Work out the finished part from the listing and answer in its coordinate system (mm). Face numbers are marked on the shaded views. Round coordinates to 2 decimals unless told otherwise and drop trailing zeros. Order: outer loops, then holes, each group sorted by start corner. A loop starts at its lowest first (then second) coordinate and runs counter-clockwise, first axis right, second up. Notation, with made-up numbers: M 76.25,20.25 L 92.25,20.25 A23 ccw 92.25,45.25 Z; hole C 14.5,-25 d10. An arc over 180 degrees is marked long. Return JSON: item names as keys, results as strings.
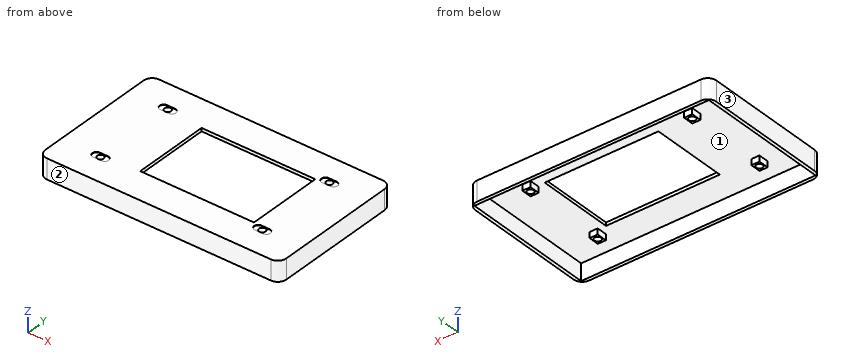
Autodesk Inventor part; units mm, degrees
ref_plane "Work Plane4" through (92.935, -15.405, 0) normal (0, 0, 1) x (1, 0, 0)
ref_plane "Work Plane5" through (-62.51, -33.015, -8.55) normal (0, 0, 1) x (1, 0, 0)
ref_plane "YZ Plane" through (0, 0, 0) normal (1, 0, 0) x (0, 1, 0)
ref_plane "Work Plane3" through (32.97, 21.365, 7.071) normal (0, 0, 1) x (1, 0, 0)
sketch "Sketch3" plane through (32.97, 21.365, 7.071) normal (0, 0, 1) x (1, 0, 0)
  line L0 (93.98, -54.61) -> (-93.98, -54.61)
  line L1 (-93.98, -54.61) -> (-93.98, 54.61)
  line L2 (-93.98, 54.61) -> (93.98, 54.61)
  line L3 (93.98, 54.61) -> (93.98, -54.61)
  line L4 (93.98, -54.61) -> (-93.98, 54.61) construction
  line L5 (-93.98, -54.61) -> (93.98, 54.61) construction
  line L6 (83.1, 48.8) -> (83.1, -50.3)
  line L7 (-81.6, 50.3) -> (81.6, 50.3)
  line L8 (-32.5, -25) -> (-32.5, 25)
  line L9 (52.4242, 25) -> (52.4242, -25)
  line L10 (49.4242, -28) -> (-29.5, -28)
  line L11 (-29.5, 28) -> (49.4242, 28)
  line L12 (-34.405, 29.905) -> (54.3292, 29.905)
  line L13 (54.3292, 29.905) -> (54.3292, -29.905)
  line L14 (54.3292, -29.905) -> (-34.405, -29.905)
  line L15 (-34.405, -29.905) -> (-34.405, 29.905)
  line L16 (49.4242, 28) -> (-29.5, 28)
  line L17 (-32.5, 25) -> (-32.5, -25)
  line L18 (49.4242, -28) -> (-29.5, -28)
  point P0 (-56.9284, 33.08)
  dimension "d6" = 187.96
  dimension "d7" = 109.22
  dimension "d8" = 4.31
  dimension "d9" = 10.88
  dimension "d55" = 1.905
  dimension "d56" = 1.905
  dimension "d57" = 1.905
  dimension "d58" = 1.905
extrude "Extrusion2" add sketch "Sketch3" against normal blind 2.54
sketch "Sketch5" plane through (32.97, 21.365, 7.071) normal (0, 0, 1) x (1, 0, 0)
  circle A0 centre (-63.1, 32.8) radius 1.5
  circle A1 centre (-63.1, -32.8) radius 1.5
  circle A2 centre (63.1, 32.8) radius 1.5
  circle A3 centre (63.1, 32.8) radius 1.5
  circle A4 centre (63.1, 32.8) radius 1.5
  circle A5 centre (63.1, 32.8) radius 1.5
  circle A6 centre (63.1, -32.8) radius 1.5
  line L0 (-59.965, 36.77) -> (-59.965, 28.83)
  line L1 (-59.965, 36.77) -> (-66.235, 36.77)
  line L2 (-66.235, 36.77) -> (-66.235, 28.83)
  line L3 (-59.965, 28.83) -> (-66.235, 28.83)
  circle A7 centre (-63.1, 32.8) radius 1.5
  line L4 (25.03, 27.635) -> (32.97, 27.635)
  line L5 (25.03, 27.635) -> (25.03, 21.365)
  line L6 (25.03, 21.365) -> (32.97, 21.365)
  line L7 (32.97, 27.635) -> (32.97, 21.365)
  circle A8 centre (29, 24.5) radius 1.25
  line L8 (-59.965, -28.83) -> (-59.965, -36.77)
  line L9 (-59.965, -28.83) -> (-66.235, -28.83)
  line L10 (-66.235, -28.83) -> (-66.235, -36.77)
  line L11 (-59.965, -36.77) -> (-66.235, -36.77)
  circle A9 centre (-63.1, -32.8) radius 1.5
  line L12 (66.235, -28.83) -> (66.235, -36.77)
  line L13 (66.235, -28.83) -> (59.965, -28.83)
  line L14 (59.965, -28.83) -> (59.965, -36.77)
  line L15 (66.235, -36.77) -> (59.965, -36.77)
  circle A10 centre (63.1, -32.8) radius 1.5
  line L16 (66.235, 36.77) -> (66.235, 28.83)
  line L17 (66.235, 36.77) -> (59.965, 36.77)
  line L18 (59.965, 36.77) -> (59.965, 28.83)
  line L19 (66.235, 28.83) -> (59.965, 28.83)
  circle A11 centre (63.1, 32.8) radius 1.5
  point P0 (-32.97, -21.365)
sketch "Sketch4" plane through (32.97, 21.365, 7.071) normal (0, 0, 1) x (1, 0, 0)
  circle A0 centre (-63.1, 32.8) radius 1.5
  circle A1 centre (-63.1, -32.8) radius 1.5
  circle A2 centre (63.1, -32.8) radius 1.5
  circle A3 centre (63.1, 32.8) radius 1.5
  circle A4 centre (-63.1, 32.8) radius 2.54
  circle A5 centre (63.1, 32.8) radius 2.54
  circle A6 centre (-63.1, -32.8) radius 2.54
  circle A7 centre (63.1, -32.8) radius 2.54
  point P0 (-32.97, -21.365)
  dimension "d12" = 5.08
ref_plane "Work Plane4" through (92.935, -15.405, 0) normal (0, 0, 1) x (1, 0, 0)
extrude "Extrusion3" add sketch "Sketch5" against normal up to surface (7.071 mm away) contours A2 | A6 | L0 L3 L2 L1 | L8 L11 L10 L9 | L12 L15 L14 L13 | L16 L19 L18 L17
extrude "Extrusion4" cut sketch "Sketch4" against normal up to surface (7.071 mm away) contours A0 | A1 | A2 | A3 | A4 | A5 | A6 | A7
ref_plane "Work Plane5" through (-62.51, -33.015, -8.55) normal (0, 0, 1) x (1, 0, 0)
sketch "Sketch7" plane through (32.97, 21.365, 4.531) normal (0, 0, -1) x (-1, 0, 0)
  line L0 (-91.44, 52.07) -> (91.44, 52.07)
  line L1 (91.44, 52.07) -> (91.44, -52.07)
  line L2 (91.44, -52.07) -> (-91.44, -52.07)
  line L3 (-91.44, -52.07) -> (-91.44, 52.07)
  line L4 (-91.44, 52.07) -> (91.44, -52.07) construction
  line L5 (91.44, 52.07) -> (-91.44, -52.07) construction
  line L6 (-93.98, -54.61) -> (93.98, -54.61)
  line L7 (93.98, -54.61) -> (93.98, 54.61)
  line L8 (-93.98, 54.61) -> (-93.98, -54.61)
  line L9 (93.98, 54.61) -> (-93.98, 54.61)
  point P0 (32.97, -21.365)
  point P1 (0, 0)
  dimension "d22" = 2.54
  dimension "d23" = 2.54
  dimension "d24" = 2.54
  dimension "d25" = 2.54
extrude "Extrusion5" add sketch "Sketch7" along normal up to surface (13.081 mm away)
fillet "Fillet1" radius 6.63 4 edges at (-61.01, 75.975, -0.7395) (126.95, 75.975, -0.7395) (126.95, -33.245, -0.7395) (-61.01, -33.245, -0.7395)
sketch "Sketch9" plane through (32.97, 21.365, 7.071) normal (0, 0, 1) x (1, 0, 0)
  circle A0 centre (-63.1, -32.8) radius 2.54
  circle A1 centre (-63.1, 32.8) radius 2.54
  circle A2 centre (63.1, 32.8) radius 2.54
  line L0 (66.275, -32.8) -> (59.925, -32.8) construction
  circle A3 centre (63.1, -32.8) radius 2.54
  line L1 (66.275, -29.625) -> (59.925, -29.625)
  line L2 (59.925, -35.975) -> (66.275, -35.975)
  arc A4 (66.275, -35.975) -> (66.275, -29.625) centre (66.275, -32.8) ccw
  arc A5 (59.925, -29.625) -> (59.925, -35.975) centre (59.925, -32.8) ccw
  line L3 (-59.925, -32.8) -> (-66.275, -32.8) construction
  line L4 (-59.925, -29.625) -> (-66.275, -29.625)
  line L5 (-66.275, -35.975) -> (-59.925, -35.975)
  arc A6 (-59.925, -35.975) -> (-59.925, -29.625) centre (-59.925, -32.8) ccw
  arc A7 (-66.275, -29.625) -> (-66.275, -35.975) centre (-66.275, -32.8) ccw
  line L6 (66.275, 32.8) -> (59.925, 32.8) construction
  line L7 (59.965, 36.77) -> (59.965, 28.83)
  line L8 (66.275, 35.975) -> (59.925, 35.975)
  line L9 (59.925, 29.625) -> (66.275, 29.625)
  arc A8 (66.275, 29.625) -> (66.275, 35.975) centre (66.275, 32.8) ccw
  arc A9 (59.925, 35.975) -> (59.925, 29.625) centre (59.925, 32.8) ccw
  line L10 (-59.925, 32.8) -> (-66.275, 32.8) construction
  line L11 (-59.925, 35.975) -> (-66.275, 35.975)
  line L12 (-66.275, 29.625) -> (-59.925, 29.625)
  arc A10 (-59.925, 29.625) -> (-59.925, 35.975) centre (-59.925, 32.8) ccw
  arc A11 (-66.275, 35.975) -> (-66.275, 29.625) centre (-66.275, 32.8) ccw
  point P0 (-32.97, -21.365)
  dimension "d47" = 3.175
  dimension "d48" = 6.35
extrude "Extrusion6" cut sketch "Sketch9" against normal blind 0.381 contours A0 | A1 | A2 | A3 | A4 L2 A5 L1 | A6 L5 A7 L4 | L8 A8 L9 L7 | L7 L9 A9 L8 | A10 L12 A11 L11
properties part number "RPi Desk Case"
Item 1: Consider line 1 along Y through (x, z) = (-30.13, 5.5) (3 decimals); line 2 along Y through (x, z) = (-30.13, 4.5) (3 decimals); line 3 along X through (y, z) = (30.5, 1.75). Determine where each line is inside the solid, lowest interval first. Write a range as [from, to].
Output:
{"line 1": "y = [-33.245, -13.975], [-8.895, 51.625], [56.705, 75.975]", "line 2": "y = [-33.245, -30.705], [-15.405, -13.975], [-8.895, -7.465], [50.195, 51.625], [56.705, 58.135], [73.435, 75.975]", "line 3": "x = [-61.01, -58.47], [124.41, 126.95]"}
Item 2: Find section D-D (y = 63). Determine the outline of the cut face in (x, z).
Output:
{"outline": "M -61.01,-8.55 L -58.47,-8.55 L -58.47,4.53 L 124.41,4.53 L 124.41,-8.55 L 126.95,-8.55 L 126.95,7.07 L -61.01,7.07 Z"}
Item 3: Find section A-A (x = 96.07). State how many separate pieces and enclosed holes the cut face has, plus the area to 3 significant figures.
Output:
{"separate pieces": "3", "enclosed holes": "0", "area": "343 mm^2"}
Item 4: The mould has two halves that part along Y. Classify the marked faces 1, 2 and 3: pulls with the +Y half, pulls with the -Y half, needs draft (parallel to the pull), parting line crosses it, or undercut.
Output:
{"face 1": "undercut", "face 2": "pulls with the -Y half", "face 3": "needs draft"}
Item 5: Each of these flat-tipped pins is pushed along its axis until it touches: pin 1 (8 mm diameter, centred on x = 41.5, y = 63.5, fed in from -Z); pin 2 (3 mm diameter, centred on x = -31.5, y = 55, fed in from -Z); pin 3 (1.9 mm diameter, centred on x = -32, y = 55.5, fed in from +Z). Where does it stop, or does it pass through?
Output:
{"pin 1": "stops at z = 4.53", "pin 2": "stops at z = 0", "pin 3": "stops at z = 6.69"}
Item 6: Find section C-C (y = 1). Determine the outline of the cut face in (x, z) (3 decimals).
Output:
{"outline": "M -61.01,-8.55 L -58.47,-8.55 L -58.47,4.531 L -1.435,4.531 L -1.435,7.071 L -61.01,7.071 Z; M 87.299,4.531 L 124.41,4.531 L 124.41,-8.55 L 126.95,-8.55 L 126.95,7.071 L 87.299,7.071 Z"}
